```python
from build123d import *

# Parameters (mm, degrees)
F1_DEPTH      = 63.5
F1_DEPTH_BACK = 63.5
F0_W          = 25.4
F0_H          = 19.05
F2_DEPTH      = 25.4
F2_DEPTH_BACK = 25.4
F3_DEPTH      = 7.9375
F5_R          = 6.35


with BuildPart() as f1:
    # F0 (on Front) → F1 (new body, two sides)
    with BuildSketch(Plane.XZ) as f1_sk:
        Polygon((-41.275, 9.525), (-41.275, -9.525), (41.275, -9.525), (41.275, 9.525), (22.225, 9.525), align=None)
    extrude(amount=F1_DEPTH)
    extrude(f1_sk.sketch, amount=-F1_DEPTH_BACK)

    # F0 (on Front) → F2 (join, two sides)
    with BuildSketch(Plane.XZ) as f2_sk:
        with BuildLine():
            Line((22.225, 9.525), (41.275, 9.525))
            Line((41.275, 9.525), (41.275, 27.0002))
            ThreePointArc((41.275, 27.0002), (45.9246798487, 38.2255201513), (57.15, 42.8752))
            Line((57.15, 42.8752), (60.325, 42.8752))
            Line((60.325, 42.8752), (60.325, 61.9252))
            Line((60.325, 61.9252), (57.15, 61.9252))
            add(Edge.make_bspline(
                [(53.8198051539, 61.7660658354), (54.9473735192, 61.8411835235), (56.058102729, 61.8944833959), (57.15, 61.9252)],
                knots=[108.2731694202, 108.2731694202, 108.2731694202, 108.2731694202, 111.5045361635, 111.5045361635, 111.5045361635, 111.5045361635], degree=3))
            ThreePointArc((53.8198051539, 61.7660658354), (31.30369775, 50.4890119112), (22.225, 27.0002))
            Line((22.225, 27.0002), (22.225, 9.525))
        make_face()
        with Locations((73.025, 52.4002)):
            Rectangle(F0_W, F0_H)
    extrude(amount=F2_DEPTH)
    extrude(f2_sk.sketch, amount=-F2_DEPTH_BACK)

    # F0 (on Front) → F3 (join, symmetric)
    with BuildSketch(Plane.XZ):
        with BuildLine():
            add(Edge.make_bspline(
                [(-41.275, 9.525), (-40.6484546844, 32.2369696222), (16.0384543074, 59.2491029489), (53.8198051539, 61.7660658354)],
                knots=[0, 0, 0, 0, 108.2731694202, 108.2731694202, 108.2731694202, 108.2731694202], degree=3))
            Line((-41.275, 9.525), (22.225, 9.525))
            Line((22.225, 9.525), (22.225, 27.0002))
            ThreePointArc((22.225, 27.0002), (31.30369775, 50.4890119112), (53.8198051539, 61.7660658354))
        make_face()
    extrude(amount=F3_DEPTH, both=True)

    # F0 (on Front) → F4 (revolve)
    with BuildSketch(Plane.XZ):
        Polygon((85.725, 66.675), (85.725, 61.9252), (85.725, 42.8752), (85.725, 38.1), (111.125, 38.1), (111.125, 66.675), align=None)
    revolve(axis=Axis((85.725, 0, 52.3875), (0, 0, 1)))

    # F5
    f5_edges = [f1.edges().sort_by_distance(p)[0] for p in [
        (41.275, -63.5, 0),
        (-41.275, -63.5, 0),
        (-41.275, 63.5, 0),
        (41.275, 63.5, 0),
    ]]
    fillet(f5_edges, radius=F5_R)


solid = f1.part
```
Design review of the part built by this model. Coordinates are the model's own, in mm. A direction names the side the tool comes from. Coordinates: 2 decimals unless noted, no trailing zeros. Order: outer loops, then holes, each group sorted by start corner. A loop starts at its lowest first (then second) coordinate and runs counter-clockwise, first axis right, second up.
1) Take a section at A-A, the plane x = 84. Give the boundary of the cut face in (y, z) (3 decimals), and give its area (3 significant figures).
2) Mouldability with a two-part tool opening along X and no side actions: class faces 1 (the flat face through (60, 2, 42.875)), 2 (the cylindrical face through (39.464, -61.59, 0.133)), 3 (the flat face through (1, 35, 9.525)) as +X half, -X half, draft (parallel to the pull), parting line (faces both ways), or undercut.
3) Clearance check with flat-ended pins moving along their axes: pin 1 (23 mm diameter, centred on x = 70.5, y = -10, fed in from -Z); pin 2 (8 mm diameter, centred on y = -13, z = 59, fed in from +X); pin 3 (5 mm diameter, centred on x = 91.5, z = 54.5, fed in from +Y); pin 4 (3 mm diameter, centred on y = -27, z = 21, fed in from -X). State where each tip first meets the part, or that it passes through.
4) Wall thickness on line 1 along Z through (x, y) = (80.5, -19) (3 decimals); line 2 along Y through (x, z) = (32.5, 42); line 3 along Y through (x, z) = (4.5, 10): over which ranges is each line inside the solid? List them lowest first.
5) For faces 4 (the flat face through (22.225, -17, 18)), 5 (the flat face through (41.275, -1, 4)), 6 (the flat face through (22.225, 17, 18)), list the 3-axis set-ups (+Z, -Z, +X, -X, +Y, -Y) from which the entire face can be reached by the end or side of a thin tool; tool diameter is ignored.
6) Take a section at B-B, the plane y = 41.5. Give the boundary of the cut face in (x, z) (3 decimals), and give its area (3 significant figures).
Returned:
1. outline: (-25.4, 42.875) - (-25.341, 42.875) - (-25.341, 38.1) - (25.341, 38.1) - (25.341, 42.875) - (25.4, 42.875) - (25.4, 61.925) - (25.341, 61.925) - (25.341, 66.675) - (-25.341, 66.675) - (-25.341, 61.925) - (-25.4, 61.925) - close
1. area: 1,450 mm2
2. face 1: undercut
2. face 2: +X half
2. face 3: draft
3. pin 1: stops at z = 38.1
3. pin 2: stops at x = 109.48
3. pin 3: stops at y = 25.19
3. pin 4: passes through
4. line 1: z = 38.1 to 66.675
4. line 2: y = -25.4 to 25.4
4. line 3: y = -7.94 to 7.94
5. face 4: +Z, -X, -Y
5. face 5: -Z, +X, +Y, -Y
5. face 6: +Z, -X, +Y
6. outline: (-41.275, -9.525) - (41.275, -9.525) - (41.275, 9.525) - (-41.275, 9.525) - close
6. area: 1,570 mm2
